Autodesk Inventor part; units mm, degrees
ref_plane "YZ Plane" through (0, 0, 0) normal (1, 0, 0) x (0, 1, 0)
ref_plane "XZ Plane" through (0, 0, 0) normal (0, 1, 0) x (-1, 0, 0)
ref_plane "XY Plane" through (0, 0, 0) normal (0, 0, 1) x (1, 0, 0)
sketch "Sketch1" plane through (0, 0, 0) normal (0, 0, 1) x (1, 0, 0)
  arc A0 (-0.4146, 4.1159) -> (-0.7739, 3.967) centre (-0.4146, 3.6077) ccw
  line L0 (0.4146, 4.1159) -> (-0.4146, 4.1159)
  arc A1 (0.7154, 4.0255) -> (0.4146, 4.1159) centre (0.426, 3.6079) ccw
  line L1 (7.9894, -3.2484) -> (0.7154, 4.0255)
  arc A2 (7.63, -4.1159) -> (7.9894, -3.2484) centre (7.63, -3.6077) ccw
  line L2 (-7.63, -4.1159) -> (7.63, -4.1159)
  arc A3 (-7.9894, -3.2484) -> (-7.63, -4.1159) centre (-7.63, -3.6077) ccw
  line L3 (-0.7739, 3.967) -> (-7.9894, -3.2484)
  circle A4 centre (-21.0112, -2.2612) radius 2
  circle A5 centre (21.0112, -2.2612) radius 2
  arc A6 (-23.0183, 6.25) -> (-25, 4.2683) centre (-23.0183, 4.2683) ccw
  line L4 (-25, 4.2683) -> (-25, -4.2683)
  arc A7 (-25, -4.2683) -> (-23.0183, -6.25) centre (-23.0183, -4.2683) ccw
  line L5 (-23.0183, -6.25) -> (23.0183, -6.25)
  arc A8 (23.0183, -6.25) -> (25, -4.2683) centre (23.0183, -4.2683) ccw
  line L6 (25, -4.2683) -> (25, 4.2683)
  arc A9 (25, 4.2683) -> (23.0183, 6.25) centre (23.0183, 4.2683) ccw
  line L7 (23.0183, 6.25) -> (16.82, 6.25)
  arc A10 (16.82, 6.25) -> (16.82, 4.11) centre (16.82, 5.18) ccw
  line L8 (16.82, 4.11) -> (18.9356, 4.11)
  arc A11 (19.6349, 2.4086) -> (18.9356, 4.11) centre (18.9356, 3.1156) ccw
  line L9 (19.6349, 2.4086) -> (16.275, -0.9151)
  arc A12 (14.0005, -1.85) -> (16.275, -0.9151) centre (14.0005, 1.3841) ccw
  line L10 (14.0005, -1.85) -> (10.9995, -1.85)
  arc A13 (8.725, -0.9151) -> (10.9995, -1.85) centre (10.9995, 1.3841) ccw
  line L11 (8.725, -0.9151) -> (5.3651, 2.4086)
  arc A14 (6.0644, 4.11) -> (5.3651, 2.4086) centre (6.0644, 3.1156) ccw
  line L12 (6.0644, 4.11) -> (8.18, 4.11)
  arc A15 (8.18, 4.11) -> (8.18, 6.25) centre (8.18, 5.18) ccw
  line L13 (8.18, 6.25) -> (-8.18, 6.25)
  arc A16 (-8.18, 6.25) -> (-8.18, 4.11) centre (-8.18, 5.18) ccw
  line L14 (-8.18, 4.11) -> (-6.0644, 4.11)
  arc A17 (-5.3651, 2.4086) -> (-6.0644, 4.11) centre (-6.0644, 3.1156) ccw
  line L15 (-5.3651, 2.4086) -> (-8.725, -0.9151)
  arc A18 (-10.9995, -1.85) -> (-8.725, -0.9151) centre (-10.9995, 1.3841) ccw
  line L16 (-10.9995, -1.85) -> (-14.0005, -1.85)
  arc A19 (-16.275, -0.9151) -> (-14.0005, -1.85) centre (-14.0005, 1.3841) ccw
  line L17 (-16.275, -0.9151) -> (-19.6349, 2.4086)
  arc A20 (-18.9356, 4.11) -> (-19.6349, 2.4086) centre (-18.9356, 3.1156) ccw
  line L18 (-18.9356, 4.11) -> (-16.82, 4.11)
  arc A21 (-16.82, 4.11) -> (-16.82, 6.25) centre (-16.82, 5.18) ccw
  line L19 (-16.82, 6.25) -> (-23.0183, 6.25)
  point P0 (0, 0)
extrude "Extrusion1" add sketch "Sketch1" against normal blind 100
properties part number "25-5013"
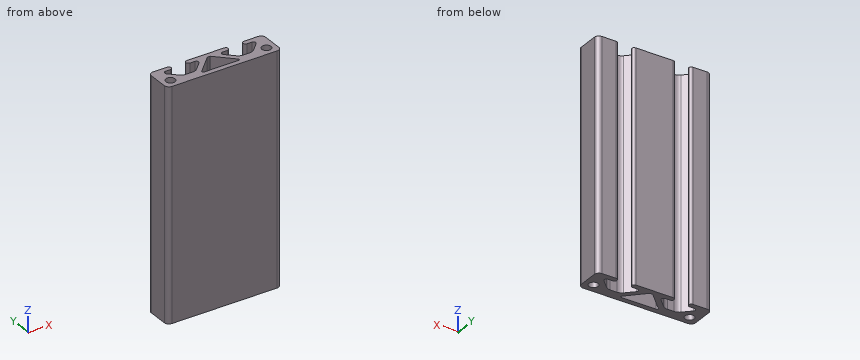
Model file for the job. Use its own axes, mm. Coordinates: 2 decimals unless noted, no trailing zeros. Order: outer loops, then holes, each group sorted by start corner. A loop starts at its lowest first (then second) coordinate and runs counter-clockwise, first axis right, second up. Notation, with made-up numbers: M -24,77.25 L 34,77.25 A32 cw 34,111.25 Z; hole C 59,7.5 d5. An arc over 180 degrees is marked long. Return JSON: item names as keys, results as strings.
1. Saw through at C-C (x = -3.5). Give the cut face in (y, z), and give its area (3 significant figures).
Ans:
{"outline": "M -6.25,-100 L -4.12,-100 L -4.12,0 L -6.25,0 Z; M 1.24,-100 L 6.25,-100 L 6.25,0 L 1.24,0 Z", "area": "714 mm^2"}
2. Saw through at D-D (z = -78). Give the number of separate pieces and of enclosed holes in the cut face, and give its area (3 significant figures).
Ans:
{"separate pieces": "1", "enclosed holes": "3", "area": "356 mm^2"}
3. Saw through at B-B (y = 5.18). Give the cut face in (x, z).
Ans:
{"outline": "M -24.78,-100 L -15.75,-100 L -15.75,0 L -24.78,0 Z; M -9.25,-100 L 9.25,-100 L 9.25,0 L -9.25,0 Z; M 15.75,-100 L 24.78,-100 L 24.78,0 L 15.75,0 Z"}
4. Flat gauge pin, fed straight in: pin 1 (0.9 mm diameter, centred on x = 13, z = -30.5, fed in from +Y). Where does the tip first touch, or does it go through?
Ans:
{"pin 1": "y = -1.85"}
5. Drill centre lines: probe 1 along X at (y, z) = (4.75, -95); probe 2 along X at (y, z) = (1, -74.5); probe 3 along X at (y, z) = (-2, -22.5). Where is each one in solid material? Low to high.
Ans:
{"probe 1": "-24.94 to -15.84, -9.16 to 9.16, 15.84 to 24.94", "probe 2": "-25 to -18.21, -6.79 to -3.74, 3.74 to 6.79, 18.21 to 25", "probe 3": "-25 to -22.99, -19.03 to -6.74, 6.74 to 19.03, 22.99 to 25"}
6. Saw through at A-A (x = -18). Give the cut face in (y, z).
Ans:
{"outline": "M -6.25,-100 L 0.79,-100 L 0.79,0 L -6.25,0 Z; M 4.11,-100 L 6.25,-100 L 6.25,0 L 4.11,0 Z"}
